from build123d import *

# Parameters (mm, degrees)
SKETCH_1_W      = 43
SKETCH_1_H      = 43
SKETCH_1_R      = 3
SKETCH_1_R_2    = 1.5
EXTRUDE_1_DEPTH = 4
SKETCH_2_R      = 3
SKETCH_2_R_2    = 1.5
EXTRUDE_2_DEPTH = 7


with BuildPart() as part:
    # 草图1 → 凸台-拉伸1 (new body)
    with BuildSketch(Plane(origin=(0, 0, 0), x_dir=(1, 0, 0), z_dir=(0, 1, 0))):
        Rectangle(SKETCH_1_W, SKETCH_1_H)
        with Locations(Location((-10, 10, 0), (0, 0, 270))):
            Circle(SKETCH_1_R, mode=Mode.SUBTRACT)
        with Locations(Location((10, 10, 0), (0, 0, 270))):
            Circle(SKETCH_1_R, mode=Mode.SUBTRACT)
        with Locations(Location((-10, -10, 0), (0, 0, 270))):
            Circle(SKETCH_1_R, mode=Mode.SUBTRACT)
        with Locations(Location((10, -10, 0), (0, 0, 270))):
            Circle(SKETCH_1_R, mode=Mode.SUBTRACT)
        with Locations(Location((-18.5, 18.5, 0), (0, 0, 270))):
            Circle(SKETCH_1_R_2, mode=Mode.SUBTRACT)
        with Locations(Location((18.5, 18.5, 0), (0, 0, 270))):
            Circle(SKETCH_1_R_2, mode=Mode.SUBTRACT)
        with Locations(Location((18.5, -18.5, 0), (0, 0, 270))):
            Circle(SKETCH_1_R_2, mode=Mode.SUBTRACT)
        with Locations(Location((-18.5, -18.5, 0), (0, 0, 270))):
            Circle(SKETCH_1_R_2, mode=Mode.SUBTRACT)
    extrude(amount=EXTRUDE_1_DEPTH)

    # 草图2 → 凸台-拉伸2 (add)
    # profile 1 of 4: a face of its own
    with BuildSketch(Plane(origin=(0, 4, 0), x_dir=(1, 0, 0), z_dir=(0, 1, 0))):
        with Locations(Location((-18.5, -18.5, 0), (0, 0, 270))):
            Circle(SKETCH_2_R)
        with Locations(Location((-18.5, -18.5, 0), (0, 0, 270))):
            Circle(SKETCH_2_R_2, mode=Mode.SUBTRACT)
    # profile 2 of 4: a face of its own
    with BuildSketch(Plane(origin=(0, 4, 0), x_dir=(1, 0, 0), z_dir=(0, 1, 0))):
        with Locations(Location((18.5, -18.5, 0), (0, 0, 270))):
            Circle(SKETCH_2_R)
        with Locations(Location((18.5, -18.5, 0), (0, 0, 270))):
            Circle(SKETCH_2_R_2, mode=Mode.SUBTRACT)
    # profile 3 of 4: a face of its own
    with BuildSketch(Plane(origin=(0, 4, 0), x_dir=(1, 0, 0), z_dir=(0, 1, 0))):
        with Locations(Location((18.5, 18.5, 0), (0, 0, 90))):
            Circle(SKETCH_2_R)
        with Locations(Location((18.5, 18.5, 0), (0, 0, 270))):
            Circle(SKETCH_2_R_2, mode=Mode.SUBTRACT)
    # profile 4 of 4: a face of its own
    with BuildSketch(Plane(origin=(0, 4, 0), x_dir=(1, 0, 0), z_dir=(0, 1, 0))):
        with Locations(Location((-18.5, 18.5, 0), (0, 0, 90))):
            Circle(SKETCH_2_R)
        with Locations(Location((-18.5, 18.5, 0), (0, 0, 270))):
            Circle(SKETCH_2_R_2, mode=Mode.SUBTRACT)
    extrude(amount=EXTRUDE_2_DEPTH)


solid = part.part
Geometry check sheet. Reference: the model listing, model coordinates, mm. A direction names the side the tool comes from. Give positions to 0.01 mm unless a question says otherwise; leave off trailing zeros. Order: outer loops, then holes, each group sorted by start corner. A loop starts at its lowest first (then second) coordinate and runs counter-clockwise, first axis right, second up.
1. Sectioned sample at C-C (z = -10). Record the boundary of the cut face in (x, y).
Completed:
outline: (-21.5, 0) - (-13, 0) - (-13, 4) - (-21.5, 4) - close; (-7, 0) - (7, 0) - (7, 4) - (-7, 4) - close; (13, 0) - (21.5, 0) - (21.5, 4) - (13, 4) - close
2. Access from +Z, -Z, +X, -X, +Y, -Y to the whole of each face (thin tool, end or side, straight path). Record for faces 1 (the face through (20, 11, -20)), 2 (the face through (21, 4, -21)), 3 (the face through (-21, 4, 21)), 4 (the face through (0, 4, 0)), 5 (the face through (-7.97, 1.97, -12.21)).
Completed:
face 1: +Z, -Z, +X, -X, +Y
face 2: -Z, +X, +Y
face 3: +Z, -X, +Y
face 4: +Y
face 5: +Y, -Y
3. Draft check along Z on faces 6 (the face through (10, 2, -13)), 7 (the face through (-17, 11, -20)), 8 (the face through (0, 2, 21.5)). Enter one of: pulls with the +Z half, pulls with the -Z half, needs draft (parallel to the pull), parting line crosses it, or undercut.
Completed:
face 6: undercut
face 7: needs draft
face 8: pulls with the +Z half
4. Sectioned sample at D-D (y = 1.25). State how many separate pieces and enclosed holes the cut face has, then the cut area to 3 significant figures.
Completed:
separate pieces: 1
enclosed holes: 8
area: 1,710 mm2
5. Sectioned sample at B-B (x = -10). Record the boundary of the cut face in (y, z).
Completed:
outline: (0, -21.5) - (4, -21.5) - (4, -13) - (0, -13) - close; (0, -7) - (4, -7) - (4, 7) - (0, 7) - close; (0, 13) - (4, 13) - (4, 21.5) - (0, 21.5) - close
6. Scan lines: line 1 (X direction, y = 2.7, z = 10); line 2 (X direction, y = 3, z = -18.5); line 3 (Y direction, x = -7.5, z = 18). Record each from-to range of solid material in increasing order.
Completed:
line 1: x = -21.5 to -13, -7 to 7, 13 to 21.5
line 2: x = -21.5 to -20, -17 to 17, 20 to 21.5
line 3: y = 0 to 4
7. Sectioned sample at A-A (y = 10.5). Record the boundary of the cut face in (x, z), then the cut area to 3 significant figures.
Completed:
outline: circle Ø6 at (-18.5, -18.5); circle Ø6 at (-18.5, 18.5); circle Ø6 at (18.5, -18.5); circle Ø6 at (18.5, 18.5); hole circle Ø3 at (-18.5, -18.5); hole circle Ø3 at (-18.5, 18.5); hole circle Ø3 at (18.5, -18.5); hole circle Ø3 at (18.5, 18.5)
area: 84.8 mm2
8. Depth check by flat-ended pin: pin 1 (10 mm diameter, centred on x = -10, z = -2, fed in from +Y); pin 2 (3.5 mm diameter, centred on x = -10, z = 10, fed in from -Y). Enter the tip coordinate at first touch or a pass-through.
Completed:
pin 1: stops at y = 4
pin 2: passes through
